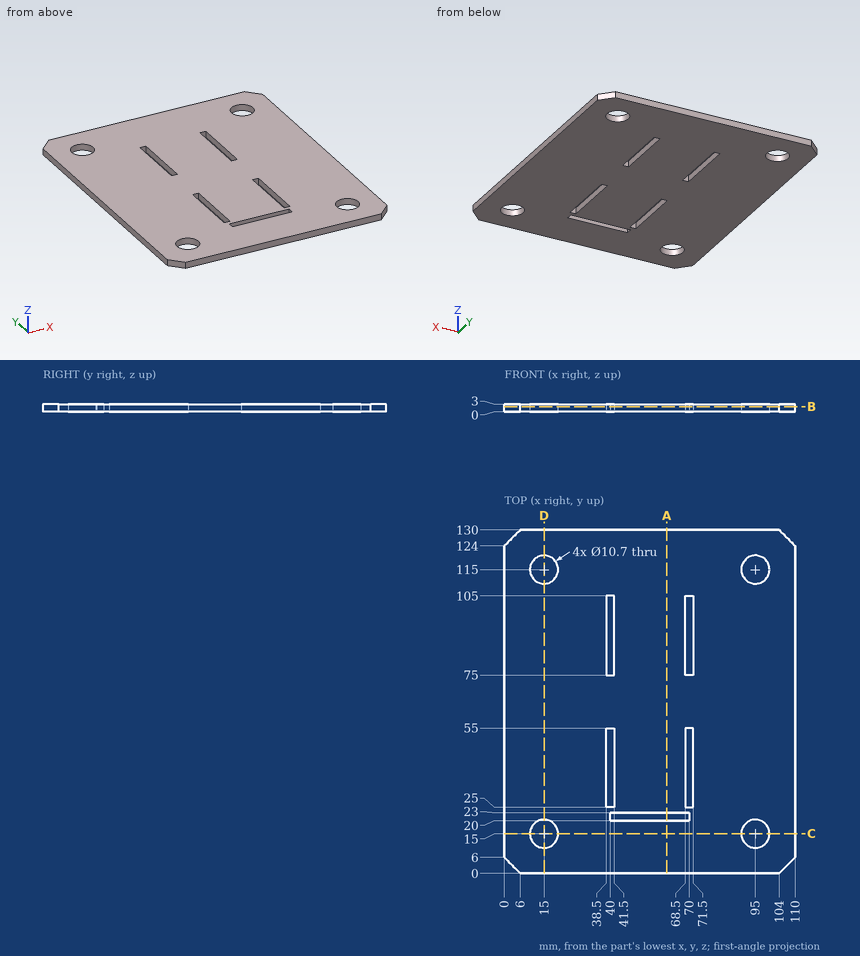
Drawing for the job (mm, zero at the part's lowest x, y, z). Round coordinates to 2 decimals unless told otherwise and drop trailing zeros. Write each loop counter-clockwise with the first axis right and the second up, starting at its lowest first coordinate (ties: lowest second). Pieces come first, ordered by that corner, then holes. Notation, with made-up numbers: (-24.75, 57.25) - (21.25, 57.25) arc R23 cw to (21.25, 84.25) - close; hole circle Ø11 at (29, 62.25). An arc over 180 degrees is marked (long way). Use CSV: the item, a comma, the result in double quotes.
(1) Band-saw the part on A-A (x = 61.5). Write the cut outline in (y, z).
Response:
outline,"(0, 0) - (20, 0) - (20, 3) - (0, 3) - close; (23, 0) - (130, 0) - (130, 3) - (23, 3) - close"
(2) Band-saw the part on B-B (z = 2). Give the number of separate pieces and of enclosed holes in the cut face, plus the area to 3 significant figures.
Response:
separate pieces,"1"
enclosed holes,"9"
area,"13,400 mm²"
(3) Band-saw the part on D-D (x = 15). Write the cut outline in (y, z), plus the area to 3 significant figures.
Response:
outline,"(0, 0) - (9.65, 0) - (9.65, 3) - (0, 3) - close; (20.35, 0) - (109.65, 0) - (109.65, 3) - (20.35, 3) - close; (120.35, 0) - (130, 0) - (130, 3) - (120.35, 3) - close"
area,"326 mm²"
(4) Wall check: line 1 (X direction, y = 38, z = 1.65); line 2 (Y direction, x = 15, z = 2.1); line 3 (X direction, y = 13, z = 2.75). Give the ranges that are in metal, low to high.
Response:
line 1,"0 to 38.5, 41.5 to 68.5, 71.5 to 110"
line 2,"0 to 9.65, 20.35 to 109.65, 120.35 to 130"
line 3,"0 to 10.04, 19.96 to 90.04, 99.96 to 110"
(5) Band-saw the part on C-C (y = 15). Write the cut outline in (x, z).
Response:
outline,"(0, 0) - (9.65, 0) - (9.65, 3) - (0, 3) - close; (20.35, 0) - (89.65, 0) - (89.65, 3) - (20.35, 3) - close; (100.35, 0) - (110, 0) - (110, 3) - (100.35, 3) - close"
